Source: three-view drawing plus pictorial views. Frame: mm from the lowest corner of the part. A direction names the side the tool comes from. Give positions to 0.01 mm unless a question says otherwise; leave off trailing zeros. Order: outer loops, then holes, each group sorted by start corner. A loop starts at its lowest first (then second) coordinate and runs counter-clockwise, first axis right, second up. Notation, with made-up numbers: (-13, 53) - (42, 53) arc R24 ccw to (42, 88) - close; hole circle Ø8 at (26, -27). An arc over 180 degrees is marked (long way). Use CSV: the item, a comma, the result in double quotes.
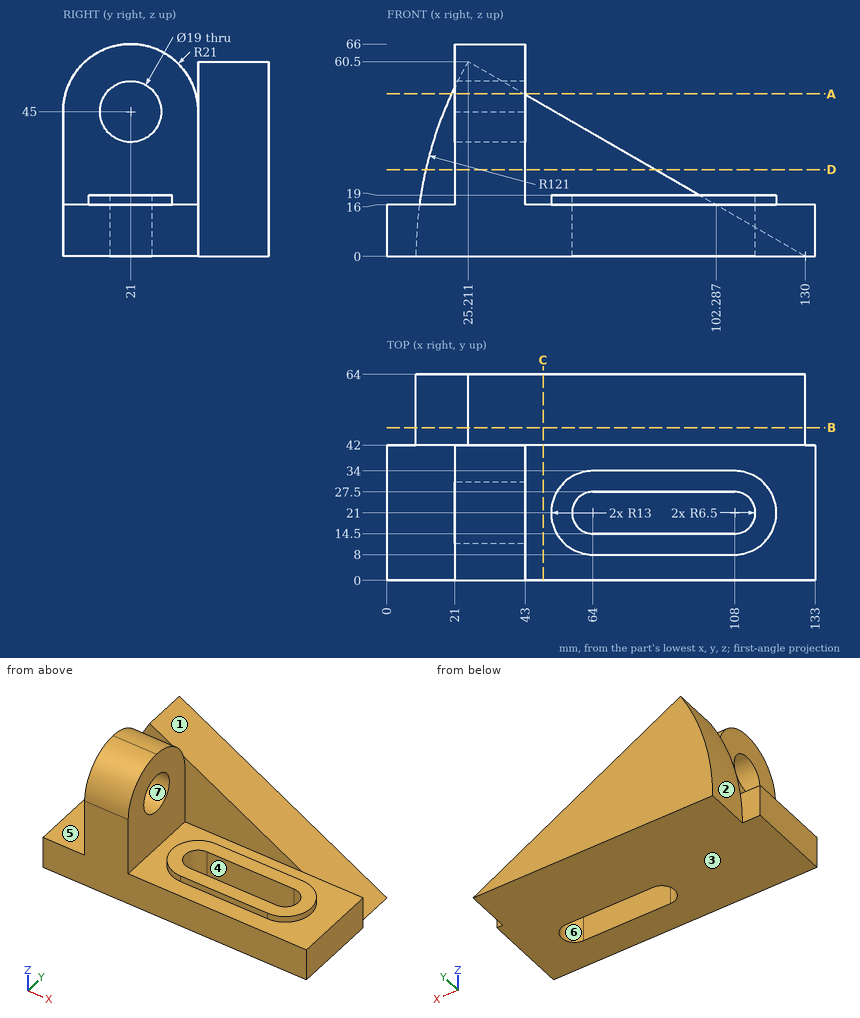
Item 1: Section C-C on x = 48.5. Return the cut outline in (y, z).
Filled in:
outline,"(0, 0) - (64, 0) - (64, 47.05) - (42, 47.05) - (42, 16) - (0, 16) - close"
Item 2: Section A-A on z = 50.5. Return the cut outline in (x, y).
Filled in:
outline,"(20.04, 42) - (42.53, 42) - (42.53, 64) - (20.04, 64) - close; (21, 0.73) - (43, 0.73) - (43, 13.25) - (21, 13.25) - close; (21, 28.75) - (43, 28.75) - (43, 41.27) - (21, 41.27) - close"
Item 3: First-contact query: pin 1 (13.5 mm diameter, centred on x = 78.5, z = 32, fed in from -Y); pin 2 (3 mm diameter, centred on x = 3.5, z = 10.5, fed in from +Y); pin 3 (21 mm diameter, centred on x = 91.5, y = 19, fed in from +Z). Flat tips, straight axial feed; report the tip coordinate or a pass-through.
Filled in:
pin 1,"stops at y = 42"
pin 2,"stops at y = 42"
pin 3,"stops at z = 19"
Item 4: Set-up query: the marked faces 5, 6 and 7. Return all of +Z, -Z, +X, -X, +Y, -Y with unobstructed straight access to the full face (end or side cutting, diameter ignored); none if empty.
Filled in:
face 5,"+Z, -X, -Y"
face 6,"+Z, -Z"
face 7,"+X, -X"
Item 5: Section B-B on y = 47.5. Return the cut outline in (x, z).
Filled in:
outline,"(9, 0) - (130, 0) - (25.21, 60.5) arc R121 ccw to start"
Item 6: Mould query, pull axis X, two halves, no side actions, for the marked faces 1, 2, 3 and 4. Classes: released by +X, released by -X, zero draft, split by the parting line, or undercut.
Filled in:
face 1,"released by +X"
face 2,"released by -X"
face 3,"zero draft"
face 4,"undercut"
Item 7: Material intervals for line 1 (Y direction, x = 90.5, z = 18); line 2 (Y direction, x = 102, z = 15); line 3 (Z direction, x = 28, y = 21), sorted ascending. Write a range as from..to.
Filled in:
line 1,"y = 8..14.5, 27.5..34, 42..64"
line 2,"y = 0..14.5, 27.5..64"
line 3,"z = 0..35.5, 54.5..66"
Item 8: Section D-D on z = 27. Return the cut outline in (x, y) (1 decimal), then the cut area to 3 significant figures.
Filled in:
outline,"(12.1, 42) - (21, 42) - (21, 0) - (43, 0) - (43, 42) - (83.2, 42) - (83.2, 64) - (12.1, 64) - close"
area,"2,490 mm2"
